Design review of the part built by this model. Coordinates are the model's own, in mm. A direction names the side the tool comes from. Coordinates: 2 decimals unless noted, no trailing zeros. Order: outer loops, then holes, each group sorted by start corner. A loop starts at its lowest first (then second) coordinate and runs counter-clockwise, first axis right, second up. Notation, with made-up numbers: (-6.5, -18) -> (26.5, -18) arc R13 ccw to (26.5, -9) -> close; hole circle Ø3 at (48, 61). An arc over 180 degrees is marked (long way). Use a Markdown table: item, result. Add a question column.
Q1. Add section D-D (z = 3.25). State the section outline as (x, y) points, then the cut area to 3 significant figures.
Q2. Add section B-B (z = 7). State the section outline as (x, y) points.
Q3. Wall thickness on probe 1 along Y at (x, z) = (0, 1.6); probe 2 along Z at (x, y) = (0, -6.95); probe 3 along X at (y, z) = (2, 12.5): over which ranges is each line inside the solid? List them lowest first.
Q4. Machinability: for faces 1 (the face through (-0.17, 8.15, 8.21)), 2 (the face through (-2.222, -10.006, 9.937)), which of the approach directions +Z, -Z, +X, -X, +Y, -Y give a long, thin tool a straight path to every point of the face, cutting with its end or side? Answer none if there is none.
Q5. Add section A-A (y = 0). State the section outline as (x, z) points.
Q6. Add section C-C (z = 9.5). State the section outline as (x, y) points.
Q7. The part is to be moulded in two halves that separate along X. For faces 3 (the face through (-0.17, 14.29, 2.46)), 4 (the face through (7, 0, 0)), 5 (the face through (-3.47, -15.62, 2.22)), say which applies: pulls with the +X half, pulls with the -X half, needs draft (parallel to the pull), parting line crosses it, or undercut.
Q8. Insertion check: pin 1 (3 mm diameter, centred on x = 0, z = 9.5, fed in from -Y); pin 2 (4 mm diameter, centred on y = 1, z = 6.5, fed in from +X); pin 3 (4 mm diameter, centred on x = -13, y = 0, fed in from +Z). Each pin has a flat end and moves straight along its axis. Give the tip position at first contact, or say it passes through.
from build123d import *

# Parameters (mm, degrees)
SKETCH1_R               = 16
SKETCH1_R_2             = 1.3
SKETCH1_R_3             = 6.25
BOSS_EXTRUDE1_DEPTH     = 5
SKETCH3_R               = 10.25
SKETCH3_R_2             = 6.25
BOSS_EXTRUDE2_DEPTH     = 15
SKETCH4_R               = 1.3
CUT_EXTRUDE5_DEPTH      = 17
CUT_EXTRUDE5_DEPTH_BACK = 17
FILLET1_R               = 0.5


with BuildPart() as part:
    # Sketch1 → Boss-Extrude1 (new body)
    with BuildSketch(Plane.XY):
        Circle(SKETCH1_R)
        with Locations((0, 13)):
            Circle(SKETCH1_R_2, mode=Mode.SUBTRACT)
        with Locations((13, 0)):
            Circle(SKETCH1_R_2, mode=Mode.SUBTRACT)
        with Locations((0, -13)):
            Circle(SKETCH1_R_2, mode=Mode.SUBTRACT)
        with Locations((-13, 0)):
            Circle(SKETCH1_R_2, mode=Mode.SUBTRACT)
        Circle(SKETCH1_R_3, mode=Mode.SUBTRACT)
    extrude(amount=BOSS_EXTRUDE1_DEPTH)

    # Sketch3 → Boss-Extrude2 (add)
    with BuildSketch(Plane.XY):
        Circle(SKETCH3_R)
        Circle(SKETCH3_R_2, mode=Mode.SUBTRACT)
    extrude(amount=BOSS_EXTRUDE2_DEPTH)

    # Sketch4 → Cut-Extrude5 (cut, two sides)
    with BuildSketch(Plane(origin=(0, 0, 0), x_dir=(1, 0, 0), z_dir=(0, 1, 0))) as cut_extrude5_sk:
        with Locations((0, -9.5)):
            Circle(SKETCH4_R)
    extrude(amount=CUT_EXTRUDE5_DEPTH, mode=Mode.SUBTRACT)
    extrude(cut_extrude5_sk.sketch, amount=-CUT_EXTRUDE5_DEPTH_BACK, mode=Mode.SUBTRACT)

    # Fillet1
    fillet1_edges = [part.edges().sort_by_distance(p)[0] for p in [
        (-10.25, 0, 5),
        (-10.25, 0, 15),
        (-16, 0, 5),
    ]]
    fillet(fillet1_edges, radius=FILLET1_R)


solid = part.part
Established:
| question | item | result |
|---|---|---|
| 1 | outline | circle Ø32 at (0, 0); hole circle Ø2.6 at (-13, 0); hole circle Ø12.5 at (0, 0); hole circle Ø2.6 at (0, -13); hole circle Ø2.6 at (0, 13); hole circle Ø2.6 at (13, 0) |
| 1 | area | 660 mm^2 |
| 2 | outline | circle Ø20.5 at (0, 0); hole circle Ø12.5 at (0, 0) |
| 3 | probe 1 | -16 to -14.3, -11.7 to -6.25, 6.25 to 11.7, 14.3 to 16 |
| 3 | probe 2 | 0 to 8.2, 10.8 to 15 |
| 3 | probe 3 | -10.05 to -5.92, 5.92 to 10.05 |
| 4 | face 1 | +Y, -Y |
| 4 | face 2 | +Z |
| 5 | outline | (-16, 0) -> (-14.3, 0) -> (-14.3, 5) -> (-15.5, 5) arc R0.5 ccw to (-16, 4.5) -> close; (-11.7, 0) -> (-6.25, 0) -> (-6.25, 15) -> (-9.75, 15) arc R0.5 ccw to (-10.25, 14.5) -> (-10.25, 5.5) arc R0.5 cw to (-10.75, 5) -> (-11.7, 5) -> close; (6.25, 0) -> (11.7, 0) -> (11.7, 5) -> (10.75, 5) arc R0.5 cw to (10.25, 5.5) -> (10.25, 14.5) arc R0.5 ccw to (9.75, 15) -> (6.25, 15) -> close; (14.3, 0) -> (16, 0) -> (16, 4.5) arc R0.5 ccw to (15.5, 5) -> (14.3, 5) -> close |
| 6 | outline | (-1.3, -10.17) -> (-1.3, -6.11) arc R6.25 cw to (-1.3, 6.11) -> (-1.3, 10.17) arc R10.25 ccw to start; (1.3, -10.17) arc R10.25 ccw to (1.3, 10.17) -> (1.3, 6.11) arc R6.25 cw to (1.3, -6.11) -> close |
| 7 | face 3 | undercut |
| 7 | face 4 | needs draft |
| 7 | face 5 | parting line crosses it |
| 8 | pin 1 | y = -10.25 |
| 8 | pin 2 | x = 15.99 |
| 8 | pin 3 | z = 5 |
